Autodesk Fusion 360 part; units mm, degrees
sketch "Boceto1" plane through (0, 0, 0) normal (0, 0, 1) x (1, 0, 0)
  circle A0 centre (0, 0) radius 10.5
  dimension "d1" = 21
extrude "Extruir1" add sketch "Boceto1" along normal blind 40
sketch "Boceto2" plane through (0, 0, 40) normal (0, 0, 1) x (-1, 0, 0)
  circle A0 centre (0, 0) radius 10.5
  circle A1 centre (0, 0) radius 20
  line L0 (20, 0) -> (-80, 0)
  circle A2 centre (-70, 0) radius 10
  line L1 (0, -20) -> (-70, -10)
  line L2 (-70, 10) -> (0, 20)
  dimension "d4" = 40
  dimension "d5" = 100
extrude "Extruir2" add sketch "Boceto2" along normal blind 20 contours A0 L0 | A0 A1 L0 L1 | A0 A1 L0 L2 | A0 L0 | A1 L0 A2 L2 | A1 L0 A2 L1 | L0 A2 | L0 A2

Autodesk Fusion 360 part; units mm, degrees
sketch "Boceto1" plane through (0, 0, 0) normal (0, 0, 1) x (1, 0, 0)
  line L0 (0, 0) -> (100, 0)
  line L1 (100, 0) -> (100, 30)
  line L2 (100, 30) -> (0, 30)
  line L3 (0, 30) -> (0, 0)
  circle A0 centre (20, 15) radius 10.5
  dimension "d1" = 100
  dimension "d2" = 30
  dimension "d3" = 21
extrude "Extruir1" add sketch "Boceto1" along normal blind 20
CAD build for the part. Positions are in the model's coordinates, mm. A direction names the side the tool comes from. Give positions to 0.01 mm unless a question says otherwise; leave off trailing zeros. Loops run counter-clockwise (first coordinate to the right, second up) from the corner with the lowest first, then second, coordinate; pieces in that order, holes last. Notation, with made-up numbers: M 5.25,50.5 L 54.25,50.5 A32 ccw 54.25,83.5 Z; hole C 11,66.5 d5. An arc over 180 degrees is marked long. One line per question, with ' | ' between items. Start each with the question number.
1. Two-plate mould, pull along X, no slides. Class faces 5 (the face through (24.845, 24.315, 19.72)), 6 (the face through (49, 15, 0)), 7 (the face through (0, 15, 20)): pulls with the +X half, pulls with the -X half, needs draft (parallel to the pull), parting line crosses it, or undercut.
2. 3-axis set-ups, long thin cutter, end or side, ignore diameter. For faces 1 (the face through (49, 0, 20)), 2 (the face through (60, 19, 40)), 3 (the face through (-20, 0, 50)), 4 (the face through (80, 0, 50)): which of +Z, -Z, +X, -X, +Y, -Y reach the whole face in a straight line?
3. Saw through at B-B on z = 33. Give the cut face in (x, y), plus the area to 3 significant figures.
4. Saw through at A-A on x = 20. Give the cut face in (y, z).
5. Flat gauge pins, fed straight in: pin 1 (12 mm diameter, centred on y = 22.5, z = 23, fed in from -X); pin 2 (4 mm diameter, centred on x = 24.5, y = 12.5, fed in from -Z); pin 3 (5 mm diameter, centred on x = 61.5, z = 6.5, fed in from -Y). Where does each tip first touch, or does it go through?
6. Probe L1, parallel to Y at x = 20, z = 17; L2, parallel to Y at x = 81.5, z = 4; L3, parallel to X at y = 15, z = 13. List the from-to ranges inside material, lowest first. Write a range as from..to.
7. Saw through at D-D on x = 90.5. Give the cut face in (y, z), plus the area to 3 significant figures.
8. Saw through at C-C on y = 2.5. Give the cut face in (x, z), plus the area to 3 significant figures.
Result sheet:
1) face 5: undercut | face 6: needs draft | face 7: pulls with the -X half
2) face 1: -Z, +X, -X, -Y | face 2: +Z, +X, +Y | face 3: +Z, -Z, -X | face 4: +Z, +X
3) outline: M 0,0 L 100,0 L 100,30 L 0,30 Z; hole C 20,15 d21 | area: 2,650 mm^2
4) outline: M -17.14,40 L 0,40 L 0,0 L 4.5,0 L 4.5,40 L 17.14,40 L 17.14,60 L -17.14,60 Z; M 25.5,0 L 30,0 L 30,40 L 25.5,40 Z
5) pin 1: stops at x = 0 | pin 2: stops at z = 40 | pin 3: stops at y = 0
6) L1: y = 0..4.5, 25.5..30 | L2: y = 0..30 | L3: x = 0..9.5, 30.5..100
7) outline: M 0,0 L 30,0 L 30,40 L 0,40 Z | area: 1,200 mm^2
8) outline: M -19.84,40 L 0,40 L 0,0 L 100,0 L 100,40 L 79.68,40 L 79.68,60 L -19.84,60 Z | area: 5,990 mm^2
